Can you work these out from the model? Positions are in its coordinate system, mm. A direction names the side the tool comes from. Give positions to 0.01 mm unless a question says otherwise; leave off trailing zeros. Order: outer loops, then holes, each group sorted by start corner. A loop starts at its lowest first (then second) coordinate and runs counter-clockwise, first axis right, second up. Notation, with made-up numbers: (-26.75, -20) - (21.25, -20) arc R18 cw to (21.25, 5) - close; hole circle Ø3 at (-2.5, 66.25). An arc over 180 degrees is marked (long way). One line per question, with ' | ' between items.
```python
from build123d import *

# Parameters (mm, degrees)
F0_R      = 66.359491572
F1_DEPTH  = 101.6
F2_DEPTH  = 25.4
F3_W      = 9.6355099231
F3_H      = 53.5687487572
F4_DEPTH  = 635
F5_DEPTH  = 25.4
F9_DEPTH  = 25.4
F10_R     = 44.5685010644
F11_DEPTH = 25.4


# Not quite as in the source:
# - the program builds the solid bodies; features that only make, move or delete a surface that nothing else refers to are left out


with BuildPart() as f1:
    # F0 (on Top) → F1 (new body)
    with BuildSketch(Plane.XY):
        Circle(F0_R)
    extrude(amount=F1_DEPTH)

    # F2 (add): a face of the model
    f2_faces = [f1.faces().sort_by_distance(p)[0] for p in [
        (0, 0, 101.6),
    ]]
    extrude(f2_faces, amount=F2_DEPTH)

    # F3 (on face) → F4 (join)
    with BuildSketch(Plane.XY.offset(127)):
        with Locations((4.8177549616, -5.3717447445)):
            Rectangle(F3_W, F3_H)
    extrude(amount=F4_DEPTH)

    # F5 (add): a face of the model
    f5_faces = [f1.faces().sort_by_distance(p)[0] for p in [
        (0, -5.3717447445, 444.5),
    ]]
    extrude(f5_faces, amount=F5_DEPTH)

    # F8 (on face) → F9 (cut)
    with BuildSketch(Plane(origin=(-25.4, 0, 0), x_dir=(0, -1, 0), z_dir=(-1, 0, 0))):
        with BuildLine():
            Line((-21.4126296341, 762), (-21.4126296341, 601.4327447423))
            ThreePointArc((-21.4126296341, 601.4327447423), (5.5404234134, 599.4593595949), (32.1561191231, 604.1461558799))
            Line((32.1561191231, 604.1461558799), (32.1561191231, 762))
            Line((32.1561191231, 762), (-21.4126296341, 762))
        make_face()
        with BuildLine():
            ThreePointArc((32.1561191231, 604.1461558799), (88.0808871948, 643.7512740199), (109.5204650209, 708.8395953178))
            ThreePointArc((109.5204650209, 708.8395953178), (-69.4608202642, 793.5150150489), (-21.4126296341, 601.4327447423))
            Line((-21.4126296341, 601.4327447423), (-21.4126296341, 762))
            Line((-21.4126296341, 762), (32.1561191231, 762))
            Line((32.1561191231, 762), (32.1561191231, 604.1461558799))
        make_face()
    extrude(amount=-F9_DEPTH, mode=Mode.SUBTRACT)

    # F10 (on Front) → F11 (cut)
    with BuildSketch(Plane.XZ):
        with Locations((0, 261.4895105362)):
            Circle(F10_R)
    extrude(amount=-F11_DEPTH, mode=Mode.SUBTRACT)


solid = f1.part
```
(1) Imagine slicing it at A-A (y = -21.5). List the corners of the cut face in (x, z) for me, and give its area (3 significant figures).
Answer below:
outline: (-62.78, 0) - (62.78, 0) - (62.78, 127) - (9.64, 127) - (9.64, 762) - (0, 762) - (0, 601.45) - (-25.4, 601.45) - (-25.4, 127) - (-62.78, 127) - close | area: 34,100 mm^2
(2) On a 3-axis mill with a long thin cutter (end or side, diameter ignored), from which of +Z, -Z, +X, -X, +Y, -Y can I reach the whole of each face in a straight line? I mean faces 1 (the face through (9.636, -6, 440)), 2 (the face through (-8, 21.413, 475)), 3 (the face through (-8.35, 10.56, 305.27)). Say none if no direction works.
Answer below:
face 1: +Z, +X, +Y, -Y | face 2: +Z, +X, -X, +Y | face 3: +Y
(3) If we mould it in two halves opening along Y, with no side actions, what happens to faces 4 (the face through (-8, 0, 262)), 5 (the face through (-14.39, -64.78, 62.61)), 6 (the face through (-12.88, -5.16, 599.44)), 7 (the face through (-25.4, -6, 362))? For each: released by +Y, released by -Y, zero draft, split by the parting line, or undercut.
Answer below:
face 4: released by +Y | face 5: split by the parting line | face 6: undercut | face 7: zero draft
(4) If I drill on line 1 (Y direction, x = -23.5, z = 558.5); line 2 (X direction, y = -6.5, z = 719.5); line 3 (Z direction, x = 27, y = -5.5), over which ranges is the centre line in solid material (lowest first)?
Answer below:
line 1: -32.16 to 21.41 | line 2: 0 to 9.64 | line 3: 0 to 127
(5) Will these pins go through, and if not, where does the flat tip stop? pin 1 (1 mm diameter, centred on x = 27.5, y = 2, fed in from -Z); pin 2 (10 mm diameter, centred on y = -34, z = 438, fed in from -X); pin 3 (10 mm diameter, centred on y = 24.5, z = 408, fed in from +X); pin 4 (10.5 mm diameter, centred on x = -10.5, z = 418, fed in from +Y).
Answer below:
pin 1: z = 0 | pin 2: x = -25.4 | pin 3: x = 9.64 | pin 4: y = 21.41
(6) Imagine slicing it at C-C (x = -51.5). List the corners of the cut face in (y, z) for me.
Answer below:
outline: (-41.85, 0) - (41.85, 0) - (41.85, 127) - (-41.85, 127) - close
(7) Imagine slicing it at B-B (z = 650). List the corners of the cut face in (x, y) for me, and give its area (3 significant figures).
Answer below:
outline: (0, -32.16) - (9.64, -32.16) - (9.64, 21.41) - (0, 21.41) - close | area: 516 mm^2
